Build history of the part. All positions in model axes, mm. Face numbers are marked on the shaded views. A direction names the side the tool comes from. Coordinates: 2 decimals unless noted, no trailing zeros. Write each loop counter-clockwise with the first axis right and the second up, starting at its lowest first coordinate (ties: lowest second). Pieces come first, ordered by that corner, then holes.
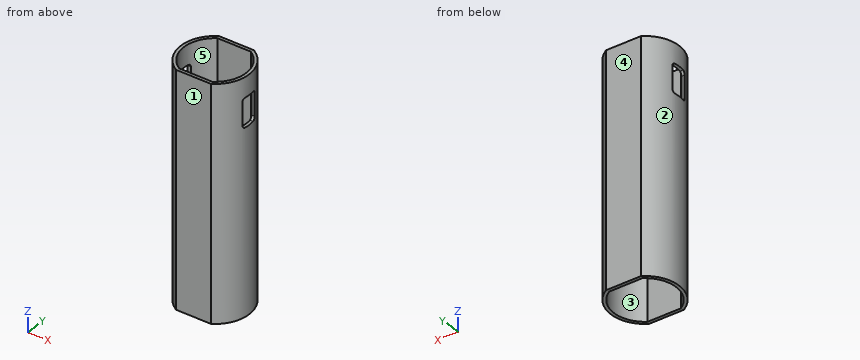
from build123d import *

# Parameters (mm, degrees)
BOSS_EXTRUDE1_DEPTH     = 150
CUT_EXTRUDE1_DEPTH      = 23
CUT_EXTRUDE1_DEPTH_BACK = 23
SCALE1_SCALE            = 0.5


with BuildPart() as part:
    # Sketch1 → Boss-Extrude1 (new body)
    with BuildSketch(Plane.XY):
        with BuildLine():
            Line((11.090536506, 19), (-11.090536506, 19))
            ThreePointArc((-11.090536506, 19), (-22, 0), (-11.090536506, -19))
            Line((-11.090536506, -19), (11.090536506, -19))
            ThreePointArc((11.090536506, -19), (22, 0), (11.090536506, 19))
        make_face()
        with BuildLine():
            Line((10.535653753, 17), (-10.535653753, 17))
            ThreePointArc((-10.535653753, 17), (-20, 0), (-10.535653753, -17))
            Line((-10.535653753, -17), (10.535653753, -17))
            ThreePointArc((10.535653753, -17), (20, 0), (10.535653753, 17))
        make_face(mode=Mode.SUBTRACT)
    extrude(amount=BOSS_EXTRUDE1_DEPTH)

    # Sketch2 → Cut-Extrude1 (cut, two sides)
    with BuildSketch(Plane(origin=(0, 0, 0), x_dir=(0, 0, -1), z_dir=(1, 0, 0))) as cut_extrude1_sk:
        with BuildLine():
            Line((-135.063632734, 5.44778031), (-120.375877862, 5.44778031))
            ThreePointArc((-120.375877862, 5.44778031), (-118.961664299, 4.861993873), (-118.375877862, 3.44778031))
            Line((-118.375877862, 3.44778031), (-118.375877862, -3.44778031))
            ThreePointArc((-118.375877862, -3.44778031), (-118.961664299, -4.861993873), (-120.375877862, -5.44778031))
            Line((-120.375877862, -5.44778031), (-135.063632734, -5.44778031))
            ThreePointArc((-135.063632734, -5.44778031), (-136.477846296, -4.861993873), (-137.063632734, -3.44778031))
            Line((-137.063632734, -3.44778031), (-137.063632734, 3.44778031))
            ThreePointArc((-137.063632734, 3.44778031), (-136.477846296, 4.861993873), (-135.063632734, 5.44778031))
        make_face()
    extrude(amount=CUT_EXTRUDE1_DEPTH, mode=Mode.SUBTRACT)
    extrude(cut_extrude1_sk.sketch, amount=-CUT_EXTRUDE1_DEPTH_BACK, mode=Mode.SUBTRACT)


with BuildPart() as part_1:
    # Scale1: scaled about (-1.198e-06, 7.41e-07, 73.880063971)
    add(part.part.scale(SCALE1_SCALE).moved(Location((-5.99e-07, 3.7e-07, 36.940031985))))


solid = part_1.part
(1) Slice it at C-C, the plane y = -4.5. List the corners of the cut face in (x, z), and give its area (3 significant figures).
(2) Slice it at A-A, the plane x = 3.25. List the corners of the cut face in (y, z).
(3) Flat gauge pins, fed straight in: P1, Ø3, axis at x = -3, y = -5.5, coming from the -Z side; P2, Ø4, axis at y = 3, z = 62, coming from the +X side; P3, Ø1.1, axis at x = -10, z = 100, coming from the -Y side; P4, Ø1.1, axis at x = -10, z = 100, coming from the +Y side. Where does each tip first touch, or does it go through?
(4) Probe L1, parallel to Y at x = -1.5, z = 109; L2, parallel to X at y = -3.75, z = 47; L3, parallel to X at y = 1.25, z = 67. List the from-to ranges inside material, lowest first.
(5) Slice it at B-B, the plane z = 101. List the corners of the cut face in (x, y), and give its area (3 significant figures).
(6) Slice it at D-D, the plane z = 66. List the corners of the cut face in (x, y), and give its area (3 significant figures).
(7) 3-axis set-ups, long thin cutter, end or side, ignore diameter. For the marked faces 4 and 5: which of +Z, -Z, +X, -X, +Y, -Y reach the whole face in a straight line?
(8) Two-plate mould, pull along X, no slides. Class the marked faces 1, 2 and 3: pulls with the +X half, pulls with the -X half, needs draft (parallel to the pull), parting line crosses it, or undercut.
Results:
1. outline: (-10.04, 36.94) - (-8.93, 36.94) - (-8.93, 111.94) - (-10.04, 111.94) - close; (8.93, 36.94) - (10.04, 36.94) - (10.04, 111.94) - (8.93, 111.94) - close
1. area: 166 mm2
2. outline: (-9.5, 36.94) - (-8.5, 36.94) - (-8.5, 111.94) - (-9.5, 111.94) - close; (8.5, 36.94) - (9.5, 36.94) - (9.5, 111.94) - (8.5, 111.94) - close
3. P1: passes through
3. P2: stops at x = 10.95
3. P3: stops at y = -5.63
3. P4: stops at y = 5.63
4. L1: y = -9.5 to -8.5, 8.5 to 9.5
4. L2: x = -10.34 to -9.27, 9.27 to 10.34
4. L3: x = -10.93 to -9.92, 9.92 to 10.93
5. outline: (-10.66, -2.72) arc R11 ccw to (-5.55, -9.5) - (5.55, -9.5) arc R11 ccw to (10.66, -2.72) - (9.62, -2.72) arc R10 cw to (5.27, -8.5) - (-5.27, -8.5) arc R10 cw to (-9.62, -2.72) - close; (-10.66, 2.72) - (-9.62, 2.72) arc R10 cw to (-5.27, 8.5) - (5.27, 8.5) arc R10 cw to (9.62, 2.72) - (10.66, 2.72) arc R11 ccw to (5.55, 9.5) - (-5.55, 9.5) arc R11 ccw to start
5. area: 53.9 mm2
6. outline: (-5.55, -9.5) - (5.55, -9.5) arc R11 ccw to (5.55, 9.5) - (-5.55, 9.5) arc R11 ccw to start; hole (-5.27, -8.5) - (5.27, -8.5) arc R10 ccw to (5.27, 8.5) - (-5.27, 8.5) arc R10 ccw to start
6. area: 64.9 mm2
7. face 4: +Z, -Z, +X, -X, +Y
7. face 5: +Z, -Z
8. face 1: needs draft
8. face 2: pulls with the -X half
8. face 3: undercut
